Check sheet for the modelled part. Datum: model origin and axes. Units: mm. A direction names the side the tool comes from. Round coordinates to 2 decimals unless told otherwise and drop trailing zeros. Loops run counter-clockwise (first coordinate to the right, second up) from the corner with the lowest first, then second, coordinate; pieces in that order, holes last. Notation, with made-up numbers: (63.5, 40) -> (82.5, 40) arc R26 ccw to (82.5, 75) -> close; hole circle Ø1 at (-30, 34). An arc over 180 degrees is marked (long way). Use one line per item in the form item = value. Start each with the question number.
(1) Material ranges on probe 1 along Y at (x, z) = (12, 3.25); probe 2 along X at (y, z) = (16, 3.5); probe 3 along Y at (x, z) = (-26, 2.5), recorded low to high. Write a range as [from, to].
(2) Sectioned sample at B-B (x = -2). Record the cut outline in (y, z).
(3) Set-up check for faces 1 (the flat face through (24.385, -41, 5)), 2 (the cylindrical face through (-57.15, 56.99, 4.93)): record each of +Z, -Z, +X, -X, +Y, -Y from which the full face is reachable in a straight line by a thin tool's end or side.
(4) Sectioned sample at A-A (y = -39). Record the cut outline in (x, z), and give its area (3 significant figures).
(5) Sectioned sample at D-D (y = -19). Record the cut outline in (x, z), and give its area (3 significant figures).
(6) Draft check along X on faces 3 (the flat face through (-60, -1, 5)), 4 (the flat face through (1, -60, 5)), 5 (the flat face through (24.385, 41, 5)). Enter one of: released by +X, released by -X, zero draft, split by the parting line, or undercut.
(7) Sectioned sample at C-C (z = 5.75). Record the cut outline in (x, y).
from build123d import *

# Parameters (mm, degrees)
BOSS_EXTRUDE1_DEPTH = 10
CUT_EXTRUDE18_DEPTH = 10


with BuildPart() as part:
    # Sketch1 → Boss-Extrude1 (new body)
    with BuildSketch(Plane.XY):
        with BuildLine():
            Line((-50, 60), (50, 60))
            ThreePointArc((50, 60), (57.071067812, 57.071067812), (60, 50))
            Line((60, 50), (60, -50))
            ThreePointArc((60, -50), (57.071067812, -57.071067812), (50, -60))
            Line((50, -60), (-50, -60))
            ThreePointArc((-50, -60), (-57.071067812, -57.071067812), (-60, -50))
            Line((-60, -50), (-60, 50))
            ThreePointArc((-60, 50), (-57.071067812, 57.071067812), (-50, 60))
        make_face()
    extrude(amount=BOSS_EXTRUDE1_DEPTH)

    # Sketch2 → Cut-Extrude18 (cut)
    with BuildSketch(Plane.XY.offset(10)):
        Polygon((-29.461538462, 50), (24.384615385, 50), (24.384615385, 32.051282051), (-11.512820513, 32.051282051), (-11.512820513, 12.820512821), (24.384615385, 12.820512821), (24.384615385, -5.128205128), (-11.512820513, -5.128205128), (-11.512820513, -32.051282051), (24.384615385, -32.051282051), (24.384615385, -50), (-29.461538462, -50), align=None)
    extrude(amount=-CUT_EXTRUDE18_DEPTH, mode=Mode.SUBTRACT)


solid = part.part
Checks:
q1.probe_1 = [-60, -50], [-32.05, -5.13], [12.82, 32.05], [50, 60]
q1.probe_2 = [-60, -29.46], [-11.51, 60]
q1.probe_3 = [-60, -50], [50, 60]
q2.outline = (-60, 0) -> (-50, 0) -> (-50, 10) -> (-60, 10) -> close; (-32.05, 0) -> (-5.13, 0) -> (-5.13, 10) -> (-32.05, 10) -> close; (12.82, 0) -> (32.05, 0) -> (32.05, 10) -> (12.82, 10) -> close; (50, 0) -> (60, 0) -> (60, 10) -> (50, 10) -> close
q3.face_1 = +Z, -Z
q3.face_2 = +Z, -Z, -X, +Y
q4.outline = (-60, 0) -> (-29.46, 0) -> (-29.46, 10) -> (-60, 10) -> close; (24.38, 0) -> (60, 0) -> (60, 10) -> (24.38, 10) -> close
q4.area = 662 mm2
q5.outline = (-60, 0) -> (-29.46, 0) -> (-29.46, 10) -> (-60, 10) -> close; (-11.51, 0) -> (60, 0) -> (60, 10) -> (-11.51, 10) -> close
q5.area = 1,020 mm2
q6.face_3 = released by -X
q6.face_4 = zero draft
q6.face_5 = undercut
q7.outline = (-60, -50) arc R10 ccw to (-50, -60) -> (50, -60) arc R10 ccw to (60, -50) -> (60, 50) arc R10 ccw to (50, 60) -> (-50, 60) arc R10 ccw to (-60, 50) -> close; hole (-29.46, -50) -> (24.38, -50) -> (24.38, -32.05) -> (-11.51, -32.05) -> (-11.51, -5.13) -> (24.38, -5.13) -> (24.38, 12.82) -> (-11.51, 12.82) -> (-11.51, 32.05) -> (24.38, 32.05) -> (24.38, 50) -> (-29.46, 50) -> close
